Job drawing, mm, ordinate dimensions from the low corner. One solid piece. A direction names the side the tool comes from. Give positions to 0.01 mm unless a question says otherwise; leave off trailing zeros. Write each loop counter-clockwise with the first axis right and the second up, starting at its lowest first coordinate (ties: lowest second). Pieces come first, ordered by that corner, then holes. Notation, with made-up numbers: M -34.5,76.5 L 9.5,76.5 A28 cw 9.5,100.5 Z; hole C -27,63.5 d2. An arc over 180 degrees is marked long. Use a Markdown table: item, result.
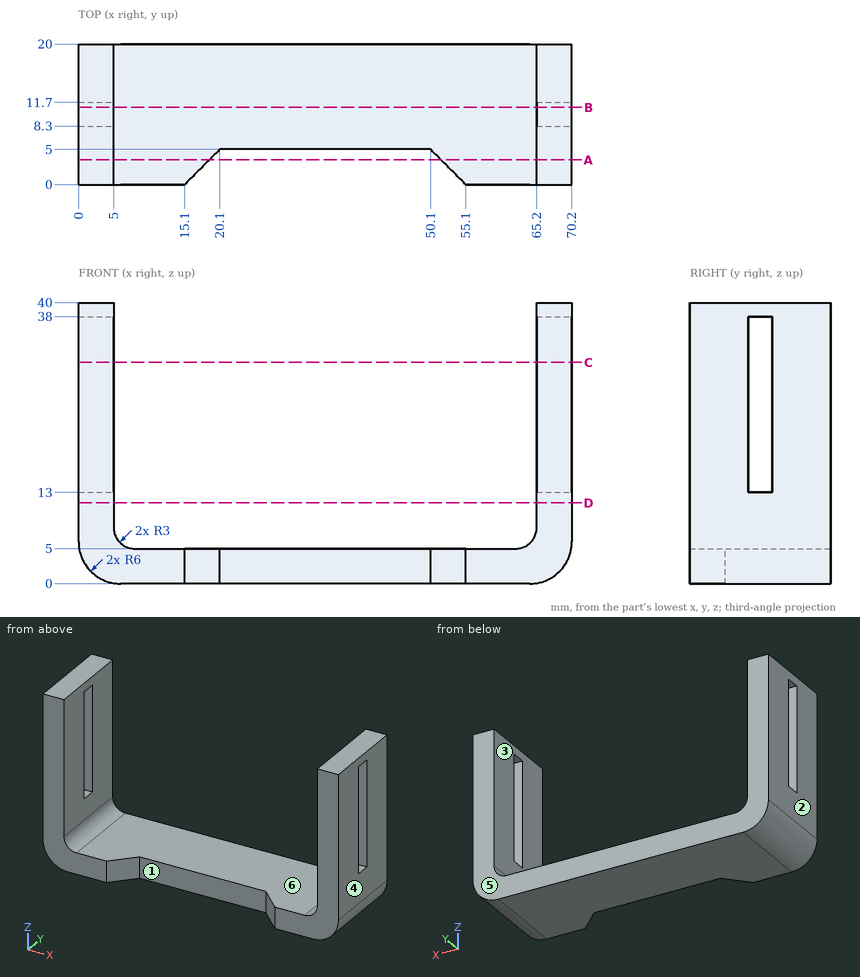
1. Cut at D-D, the plane z = 11.5. Give the cut face in (x, y).
Findings below:
| item | result |
|---|---|
| outline | M 0,0 L 5,0 L 5,20 L 0,20 Z; M 65.2,0 L 70.2,0 L 70.2,20 L 65.2,20 Z |
2. Cut at C-C, the plane z = 31.5. Give the cut face in (x, y), then the cut area to 3 significant figures.
Findings below:
| item | result |
|---|---|
| outline | M 0,0 L 5,0 L 5,8.3 L 0,8.3 Z; M 0,11.7 L 5,11.7 L 5,20 L 0,20 Z; M 65.2,0 L 70.2,0 L 70.2,8.3 L 65.2,8.3 Z; M 65.2,11.7 L 70.2,11.7 L 70.2,20 L 65.2,20 Z |
| area | 166 mm2 |
3. Cut at B-B, the plane y = 11. Give the cut face in (x, z).
Findings below:
| item | result |
|---|---|
| outline | M 0,6 A6 ccw 6,0 L 64.2,0 A6 ccw 70.2,6 L 70.2,13 L 65.2,13 L 65.2,8 A3 cw 62.2,5 L 8,5 A3 cw 5,8 L 5,13 L 0,13 Z; M 0,38 L 5,38 L 5,40 L 0,40 Z; M 65.2,38 L 70.2,38 L 70.2,40 L 65.2,40 Z |
4. Tool access for the marked faces 1, 2 and 3: list every direction of +Z, -Z, +X, -X, +Y, -Y with a clear straight run to the whole face (end or side of a thin tool).
Findings below:
| item | result |
|---|---|
| face 1 | +Z, -Z, -Y |
| face 2 | +Z, -Z, -X, +Y, -Y |
| face 3 | +Z, +Y, -Y |
5. Cut at A-A, the plane y = 3.5. Give the cut face in (x, z), then the cut area to 3 significant figures.
Findings below:
| item | result |
|---|---|
| outline | M 0,6 A6 ccw 6,0 L 18.6,0 L 18.6,5 L 8,5 A3 cw 5,8 L 5,40 L 0,40 Z; M 51.6,0 L 64.2,0 A6 ccw 70.2,6 L 70.2,40 L 65.2,40 L 65.2,8 A3 cw 62.2,5 L 51.6,5 Z |
| area | 524 mm2 |
6. Drill centre lines: L1, parallel to X at y = 3, z = 23; L2, parallel to Z at x = 57, y = 14.5; L3, parallel to Z at x = 4.5, y = 9.75. Where is each one in solid material? Low to high.
Findings below:
| item | result |
|---|---|
| L1 | 0 to 5, 65.2 to 70.2 |
| L2 | 0 to 5 |
| L3 | 0.19 to 13, 38 to 40 |
7. Two-plate mould, pull along X, no slides. Class the marked faces 4, 5 and 6: released by +X, released by -X, zero draft, split by the parting line, or undercut.
Findings below:
| item | result |
|---|---|
| face 4 | released by +X |
| face 5 | zero draft |
| face 6 | undercut |
8. Drop flat-ended pins along their axis: P1, Ø1, axis at x = 8, z = 7.5, coming from the +Y side; P2, Ø1, axis at x = 2.5, y = 10.5, coming from the -Z side; P3, Ø5.5, axis at x = 40, z = 2.5, coming from the -Y side; P4, Ø8, axis at x = 22, z = 5, coming from the -Y side. Give the stop position or say it passes through.
Findings below:
| item | result |
|---|---|
| P1 | through |
| P2 | z = 0.8 |
| P3 | y = 5 |
| P4 | y = 2.9 |
